Input: part model. Units: mm. Frame: model coordinates. Face numbers are marked on the shaded views. A direction names the side the tool comes from. Coordinates: 2 decimals unless noted, no trailing zeros. Write each loop counter-clockwise with the first axis right and the second up, starting at its lowest first coordinate (ties: lowest second). Pieces come first, ordered by that corner, then holes.
1) Line query: L1, parallel to X at y = 5, z = 5.5; L2, parallel to X at y = 5.75, z = -2.75; L3, parallel to X at y = 16.5, z = -1.25. Output: solid intervals per line, ascending.
2) Set-up query: the marked faces 4, 5 and 6. Return all of +Z, -Z, +X, -X, +Y, -Y with unobstructed straight access to the full face (end or side cutting, diameter ignored); none if empty.
3) Pin query (flat end, axial travel): pin 1 Ø0.6 at (x, y) = (-61, 10.5) entering from +Z; pin 2 Ø6 at (x, y) = (-41, 11) entering from -Z; pin 3 Ø1 at (y, z) = (12.5, 4.5) entering from -X. Return the tip coordinate at first contact, or that it passes through.
4) Section query A-A (x = -8). Output: boundary loops of the cut face in (y, z), then the cut area to 3 significant figures.
5) Section query B-B (x = 41). Output: boundary loops of the cut face in (y, z).
6) Draft query along X for the marked faces 1, 2 and 3. Return one class per face: pulls with the +X half, pulls with the -X half, needs draft (parallel to the pull), parting line crosses it, or undercut.
Autodesk Fusion 360 part; units mm, degrees
sketch "Sketch1" plane through (0, 0, 0) normal (0, 1, 0) x (1, 0, 0)
  line L0 (63.5, 7.5) -> (-63.5, 7.5)
  line L1 (-63.5, 7.5) -> (-63.5, -7.5)
  line L2 (-63.5, -7.5) -> (63.5, -7.5)
  line L3 (63.5, -7.5) -> (63.5, 7.5)
  line L4 (63.5, 7.5) -> (-63.5, -7.5) construction
  line L5 (-63.5, 7.5) -> (63.5, -7.5) construction
  line L6 (0, -7.5) -> (-14.5, -7.5) construction
  line L7 (-14.5, -7.5) -> (14.5, -7.5)
  line L8 (14.5, -7.5) -> (14.5, -2.5)
  line L9 (14.5, -2.5) -> (-14.5, -2.5)
  line L10 (-14.5, -2.5) -> (-14.5, -7.5)
  line L11 (-14.5, -2.5) -> (-18.4392, -3.1946)
  line L12 (-14.5, -2.5) -> (-11.5456, -2.5) construction
  line L13 (-14.5, -2.5) -> (-18.4392, -3.1946)
  line L14 (-18.4392, -3.1946) -> (-18.1353, -4.918)
  line L15 (-18.1353, -4.918) -> (-14.1961, -4.2234)
  line L16 (-14.1961, -4.2234) -> (-14.5, -2.5)
  line L17 (14.5, -2.5) -> (18.4392, -3.1946)
  line L18 (14.5, -2.5) -> (17.5, -2.5) construction
  line L19 (14.5, -2.5) -> (18.4392, -3.1946)
  line L20 (18.4392, -3.1946) -> (18.1353, -4.918)
  line L21 (18.1353, -4.918) -> (14.1961, -4.2234)
  line L22 (14.1961, -4.2234) -> (14.5, -2.5)
  line L23 (-63.5, 7.5) -> (-57.5, 7.5) construction
  line L24 (-57.5, 7.5) -> (-57.5, 5.5)
  line L25 (-57.5, 5.5) -> (-61.5, 5.5)
  line L26 (-61.5, 5.5) -> (-61.5, 3.75)
  line L27 (61.5, 3.7349) -> (61.5066, 5.4848)
  line L28 (61.5066, 5.4848) -> (57.5067, 5.5)
  line L29 (57.5067, 5.5) -> (57.5067, 7.5)
  line L30 (-61.5, 3.75) -> (-57.5, 3.75)
  line L31 (-57.5, 3.75) -> (-57.5, -0.25)
  line L32 (-57.5, -0.25) -> (-27.5, -0.25)
  line L33 (-27.5, -0.25) -> (-27.5, 3.75)
  line L34 (-27.5, 3.75) -> (-23.5, 3.75)
  line L35 (-23.5, 3.75) -> (-23.5, -0.25)
  line L36 (-23.5, -0.25) -> (23.5, -0.25)
  line L37 (23.5, -0.25) -> (23.5, 3.75)
  line L38 (23.5, 3.75) -> (27.5, 3.75)
  line L39 (27.5, 3.75) -> (27.5, -0.25)
  line L40 (27.5, -0.25) -> (57.5, -0.25)
  line L41 (57.5, -0.25) -> (57.5, 3.75)
  line L42 (57.5, 3.75) -> (61.5, 3.7349)
  line L43 (-61.5, 5.5) -> (-59.5, 5.5) construction
  line L44 (-60.5, 7.5) -> (-59.5, 5.5)
  line L45 (61.5066, 5.4848) -> (59.5066, 5.4924) construction
  line L46 (61.5452, 7.5) -> (59.5066, 5.4924)
  dimension "d1" = 127
  dimension "d2" = 15
  dimension "d3" = 14.5
  dimension "d5" = 29
  dimension "d6" = 5
  dimension "d7" = 190
  dimension "d8" = 4
  dimension "d9" = 1.75
  dimension "d10" = 4
  dimension "d11" = 190
  dimension "d12" = 1.75
  dimension "d15" = 6
  dimension "d16" = 2
  dimension "d17" = 4
  dimension "d18" = 1.75
  dimension "d19" = 123
  dimension "d20" = 1.75
  dimension "d21" = 4
  dimension "d22" = 2
  dimension "d23" = 4
  dimension "d24" = 4
  dimension "d25" = 30
  dimension "d26" = 4
  dimension "d27" = 4
  dimension "d28" = 47
  dimension "d29" = 4
  dimension "d30" = 4
  dimension "d31" = 4
  dimension "d32" = 30
  dimension "d33" = 4
  dimension "d38" = 89.783
extrude "Extrude3" add sketch "Sketch1" along normal blind 20 contours L0 L1 L2 L3 L8 L9 L10 L11 L13 L14 L15 L17 L19 L20 L21 L25 L26 L27 L28 L30 L31 L32 L33 L34 L35 L36 L37 L38 L39 L40 L41 L42 L44 L46
fillet "Fillet1" radius 10 2 edges at (-63.5, 10, 7.5) (63.5, 10, 7.5)
fillet "Fillet2" radius 1 6 edges at (-57.5, 10, -3.75) (-27.5, 10, -3.75) (-23.5, 10, -3.75) (23.5, 10, -3.75) (27.5, 10, -3.75) (57.5, 10, -3.75)
fillet "Fillet3" radius 1 2 edges at (-63.5, 10, -7.5) (63.5, 10, -7.5)
fillet "Fillet4" radius 2 2 edges at (-60.5, 10, -7.5) (61.5452, 10, -7.5)
fillet "Fillet5" radius 2 2 edges at (-14.5, 10, 7.5) (14.5, 10, 7.5)
equation "d3 = ( 35 / 2 ) * 1 mm - 3 mm"
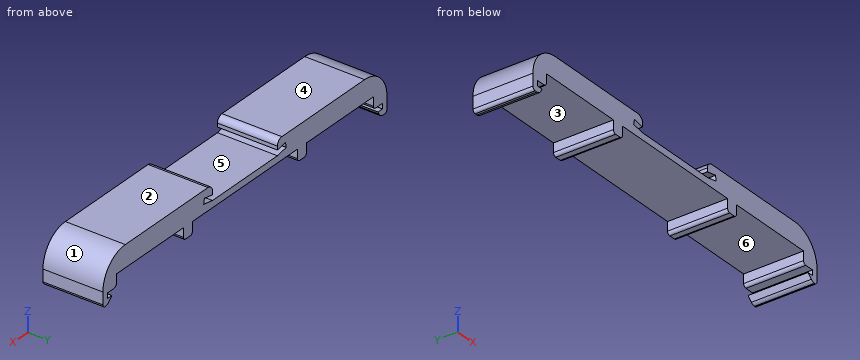
Answer:
1. L1: x = -59.5 to -14.5, 14.5 to 59.5
1. L2: x = -63.5 to -57.5, -27.5 to -23.5, 23.5 to 27.5, 57.5 to 63.5
1. L3: x = -63.42 to -57.5, -27.5 to -23.5, 23.5 to 27.5, 57.5 to 63.42
2. face 4: +Z, +X, -X, +Y, -Y
2. face 5: +Z, +Y, -Y
2. face 6: -Z, +Y, -Y
3. pin 1: stops at z = 4.44
3. pin 2: stops at z = 0.25
3. pin 3: stops at x = -61.1
4. outline: (0, 0.25) - (20, 0.25) - (20, 2.5) - (0, 2.5) - close
4. area: 45.0 mm2
5. outline: (0, 0.25) - (20, 0.25) - (20, 7.5) - (0, 7.5) - close
6. face 1: pulls with the +X half
6. face 2: needs draft
6. face 3: undercut
